Autodesk Inventor part; units mm, degrees
ref_plane "YZ Plane" through (0, 0, 0) normal (1, 0, 0) x (0, 1, 0)
ref_plane "XZ Plane" through (0, 0, 0) normal (0, 1, 0) x (-1, 0, 0)
ref_plane "XY Plane" through (0, 0, 0) normal (0, 0, 1) x (1, 0, 0)
sketch "Sketch1" plane through (0, 0, 0) normal (0, 1, 0) x (-1, 0, 0)
  line L0 (10.2, -3) -> (10.2, -46.7)
  line L1 (10.2, -46.7) -> (0.5, -46.7)
  line L2 (0.5, -46.7) -> (0.5, -45.95)
  line L3 (0.5, -45.95) -> (0, -45.95)
  line L4 (0, -45.95) -> (0, -46.7)
  line L5 (0.5, -3) -> (0.5, -3.75)
  line L6 (0.5, -3.75) -> (0, -3.75)
  line L7 (0, -3.75) -> (0, -3)
  line L8 (0, -3) -> (0, 0)
  line L9 (0, 0) -> (13.2, 0)
  line L10 (0, -49.7) -> (0, -46.7)
  line L11 (10.2, -3) -> (0.5, -3)
  line L12 (8.7, -56.4) -> (19.7, -56.4)
  line L13 (19.7, -56.4) -> (19.7, -54.7)
  line L14 (19.7, -54.7) -> (12.7, -54.7)
  line L15 (12.7, -54.7) -> (12.7, -49.7)
  line L16 (12.7, -49.7) -> (13.2, -49.7)
  line L17 (19.7, -49.7) -> (19.7, -47.45)
  line L18 (19.7, -47.45) -> (13.2, -47.45)
  line L19 (8.7, -56.4) -> (8.7, -49.7)
  arc A0 (10.2, -46.7) -> (10.2, -3) centre (-117.9506, -24.85) ccw
  line L20 (13.2, -49.7) -> (19.7, -49.7)
  line L21 (12.7, -49.7) -> (12.7, -49.7)
  line L22 (8.7, -49.7) -> (0, -49.7)
  line L23 (13.2, -47.45) -> (8.7, -49.7)
  arc A1 (13.2, -47.45) -> (13.2, 0) centre (-84.6392, -23.725) ccw
  point P0 (0, 0)
  dimension "d1" = 9.7
  dimension "d2" = 0.75
  dimension "d3" = 0.5
  dimension "d6" = 0.5
  dimension "d10" = 43.7
  dimension "d13" = 0.75
  dimension "d14" = 3
  dimension "d16" = 5
  dimension "d19" = 7
  dimension "d30" = 2.25
  dimension "d31" = 1.7
  dimension "d34" = 2.25
  dimension "d37" = 4
  dimension "d38" = 100.6746
  dimension "d39" = 130
extrude "Extrusion4" add sketch "Sketch1" along normal blind 4 contours L11 L5 L6 L7 L8 L9 A1 L23 L22 L10 L4 L3 L2 L1 A0
extrude "Extrusion5" add sketch "Sketch1" along normal blind 15 contours L23 L18 L17 L20 L16 L15 L14 L13 L12 L19
properties part number "LeftClip"
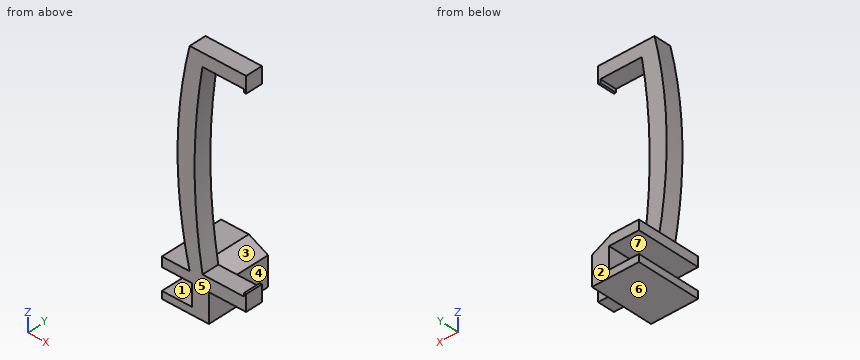
For this review, take the finished solid that the model builds, in its own axes (mm). Face numbers are marked on the shaded views. A direction names the side the tool comes from. Coordinates: 2 decimals unless noted, no trailing zeros. Loops run counter-clockwise (first coordinate to the right, second up) from the corner with the lowest first, then second, coordinate; pieces in that order, holes last.
1. Add section D-D, the plane y = 1. Give the boundary of the cut face in (x, z) (3 decimals).
2. For the marked faces 1, 2, 3 and 4, list the 3-axis set-ups (+Z, -Z, +X, -X, +Y, -Y) from which the entire face can be reached by the end or side of a thin tool; tool diameter is ignored.
3. Insertion check: P1, Ø3, axis at x = -5, y = 1.5, coming from the +Z side; P2, Ø2, axis at y = 8.5, z = -54, coming from the +X side; P3, Ø2, axis at x = -5, y = 2, coming from the -Z side. Each pin has a flat end and moves straight along its axis. Give the tip position at first contact, or say it passes through.
4. For line 1 (Z direction, x = -4.25, y = 1.5); line 2 (Y direction, x = -13.5, z = -17); line 3 (X direction, y = 5.25, z = -52.5), list the stretches that pass through material, from the lowest coordinate up.
5. Add section B-B, the plane y = 12.75. Give the boundary of the cut face in (x, z), then the cut area to 3 significant figures.
6. Add section C-C, the plane x = -17.25. Give the boundary of the cut face in (y, z).
7. Add section A-A, the plane x = -1.25. Give the boundary of the cut face in (y, z), then the cut area to 3 significant figures.
8. Mouldability with a two-part tool opening along Z and no side actions: class the marked faces 5, 6 and 7 as +Z half, -Z half, draft (parallel to the pull), parting line (faces both ways), or undercut.
Result:
1. outline: (-19.7, -56.4) - (-8.7, -56.4) - (-8.7, -49.7) - (0, -49.7) - (0, -45.95) - (-0.5, -45.95) - (-0.5, -46.7) - (-10.2, -46.7) arc R130 cw to (-10.2, -3) - (-0.5, -3) - (-0.5, -3.75) - (0, -3.75) - (0, 0) - (-13.2, 0) arc R100.675 ccw to (-13.2, -47.45) - (-19.7, -47.45) - (-19.7, -49.7) - (-12.7, -49.7) - (-12.7, -54.7) - (-19.7, -54.7) - close
2. face 1: -X, +Y, -Y
2. face 2: +Z, -Z, +X, -X, +Y
2. face 3: +Z, +X, +Y
2. face 4: -Z, +X, +Y, -Y
3. P1: stops at z = 0
3. P2: stops at x = -8.7
3. P3: stops at z = -49.7
4. line 1: z = -49.7 to -46.7, -3 to 0
4. line 2: y = 0 to 4
4. line 3: x = -12.7 to -8.7
5. outline: (-19.7, -56.4) - (-8.7, -56.4) - (-8.7, -49.7) - (-13.2, -47.45) - (-19.7, -47.45) - (-19.7, -49.7) - (-12.7, -49.7) - (-12.7, -54.7) - (-19.7, -54.7) - close
5. area: 58.4 mm2
6. outline: (0, -56.4) - (15, -56.4) - (15, -54.7) - (0, -54.7) - close; (0, -49.7) - (15, -49.7) - (15, -47.45) - (0, -47.45) - close
7. outline: (0, -49.7) - (4, -49.7) - (4, -46.7) - (0, -46.7) - close; (0, -3) - (4, -3) - (4, 0) - (0, 0) - close
7. area: 24.0 mm2
8. face 5: draft
8. face 6: -Z half
8. face 7: undercut
